from build123d import *

# Parameters (mm, degrees)
F1_DEPTH = 15
F2_R     = 2
F3_R     = 1
F4_R     = 1
F5_R     = 1


with BuildPart() as f1:
    # F0 (on Top) → F1 (new body)
    with BuildSketch(Plane.XY):
        Polygon((45.5563491861, 73.9710003696), (-40.6126983722, 73.9710003696), (-40.6126983722, 58.9710003696), (-33.5416305603, 51.8999325577), (-26.4705627485, 58.9710003696), (-13.4215728753, 45.9220104963), (-4.563708499, 45.9220104963), (8.4852813742, 58.9710003696), (15.5563491861, 51.8999325577), (3.5073593129, 39.8509426845), (3.5073593129, -52.0069216918), (15.5563491861, -64.055911565), (8.4852813742, -71.1269793769), (-4.563708499, -58.0779895037), (-13.4215728753, -58.0779895037), (-26.4705627485, -71.1269793769), (-33.5416305603, -64.055911565), (-40.6126983722, -71.1269793769), (-40.6126983722, -91.1269793769), (25.5563491861, -91.1269793769), (45.5563491861, -71.1269793769), align=None)
    extrude(amount=F1_DEPTH)

    # F2
    f2_edges = [f1.edges().sort_by_distance(p)[0] for p in [
        (-33.541631, 51.899933, 7.5),
        (-40.612698, 58.971, 7.5),
    ]]
    fillet(f2_edges, radius=F2_R)

    # F3
    f3_edges = [f1.edges().sort_by_distance(p)[0] for p in [
        (-26.470563, 58.971, 7.5),
        (-13.421573, 45.92201, 7.5),
        (-4.563708, 45.92201, 7.5),
        (8.485281, 58.971, 7.5),
        (-40.612698, 59.799427, 7.5),
    ]]
    fillet(f3_edges, radius=F3_R)

    # F4
    f4_edges = [f1.edges().sort_by_distance(p)[0] for p in [
        (-40.612698, -71.126979, 7.5),
        (-33.541631, -64.055912, 7.5),
        (-13.421573, -58.07799, 7.5),
        (-4.563708, -58.07799, 7.5),
        (15.556349, -64.055912, 7.5),
        (3.507359, -52.006922, 7.5),
        (3.507359, 39.850943, 7.5),
        (15.556349, 51.899933, 7.5),
    ]]
    fillet(f4_edges, radius=F4_R)

    # F5
    f5_edges = [f1.edges().sort_by_distance(p)[0] for p in [
        (-40.612698, 73.971, 7.5),
        (8.485281, -71.126979, 7.5),
        (-40.612698, -91.126979, 7.5),
        (45.556349, 73.971, 7.5),
        (45.556349, -71.126979, 7.5),
        (25.556349, -91.126979, 7.5),
    ]]
    fillet(f5_edges, radius=F5_R)


solid = f1.part
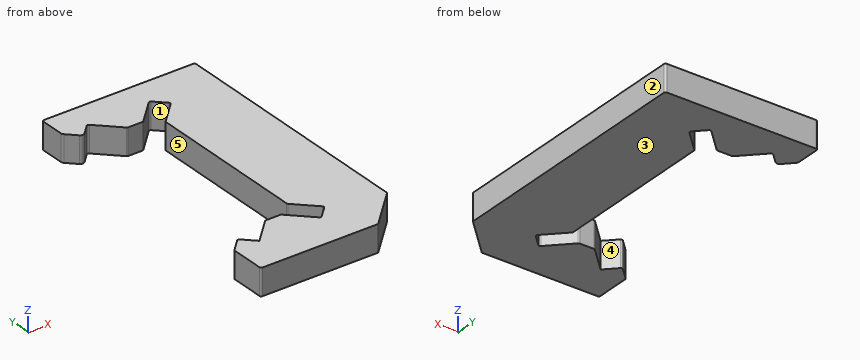
Verification items for the finished model (mm, model axes). Face numbers are marked on the shaded views. A direction names the side the tool comes from. Coordinates: 2 decimals unless noted, no trailing zeros. Loops run counter-clockwise (first coordinate to the right, second up) from the corner with the lowest first, then second, coordinate; pieces in that order, holes last. Notation, with made-up numbers: (-18, -26) -> (28, -26) arc R27 ccw to (28, 0) -> close; hole circle Ø10 at (69, 74). An arc over 180 degrees is marked (long way). Answer as a JSON object with one key per item and string values. Group by question number.
Item 1: Mould release check, pull along X, two halves, no side actions. Record for the marked faces 3, 4 and 5: +X half, -X half, draft (parallel to the pull), parting line (faces both ways), or undercut.
Item 2: Scan lines: probe 1 along Y at (x, z) = (-13, 10); probe 2 along Y at (x, z) = (-33.5, 8.5); probe 3 along X at (y, z) = (32, 1). Record each from-to range of solid material in increasing order.
Item 3: Sectioned sample at A-A on x = 6. Record the boundary of the cut face in (y, z), plus the area to 3 significant figures.
Item 4: Sectioned sample at C-C on x = 37.5. Record the boundary of the cut face in (y, z), plus the area to 3 significant figures.
Item 5: Sectioned sample at B-B on y = -31.5. Record the boundary of the cut face in (x, z), plus the area to 3 significant figures.
Item 6: Tool access check on the marked faces 1 and 2. Record the directions out of +Z, -Z, +X, -X, +Y, -Y that give a thin tool (end or side, any length) a straight path to the whole face; none if there is none.
Evaluation:
{
 "1": {"face 3": "draft", "face 4": "undercut", "face 5": "-X half"},
 "2": {"probe 1": "y = -91.13 to -58.08, 45.92 to 73.97", "probe 2": "y = -91.13 to -64.47, 52.73 to 73.97", "probe 3": "x = 3.51 to 45.56"},
 "3": {"outline": "(-91.13, 0) -> (-68.64, 0) -> (-68.64, 15) -> (-91.13, 15) -> close; (-54.5, 0) -> (42.34, 0) -> (42.34, 15) -> (-54.5, 15) -> close; (56.49, 0) -> (73.97, 0) -> (73.97, 15) -> (56.49, 15) -> close", "area": "2,050 mm²"},
 "4": {"outline": "(-79.18, 0) -> (73.97, 0) -> (73.97, 15) -> (-79.18, 15) -> close", "area": "2,300 mm²"},
 "5": {"outline": "(3.51, 0) -> (45.56, 0) -> (45.56, 15) -> (3.51, 15) -> close", "area": "631 mm²"},
 "6": {"face 1": "+Z, -Z", "face 2": "+Z, -Z, +X, +Y, -Y"}
}
